from build123d import *

# Parameters (mm, degrees)
F0_W      = 76.2
F0_H      = 76.2
F1_DEPTH  = 76.2
F2_W      = 49.722627
F2_H      = 47.354873
F3_DEPTH  = 25.4
F4_W      = 31.569913
F4_H      = 34.332275
F5_DEPTH  = 50.8
F6_W      = 22.098936
F6_H      = 25.650553
F7_DEPTH  = 154.178
F8_W      = 5.524732
F8_H      = 5.524733
F9_DEPTH  = 171.45
F10_W     = 11.54276
F10_H     = 13.466537
F11_DEPTH = 96.774


with BuildPart() as f1:
    # F0 (on Front) → F1 (new body)
    with BuildSketch(Plane.XZ):
        with Locations((-38.1, 38.1)):
            Rectangle(F0_W, F0_H)
    extrude(amount=F1_DEPTH)

    # F2 (on Top) → F3 (join)
    with BuildSketch(Plane.XY):
        with Locations((-39.363734, -40.251642)):
            Rectangle(F2_W, F2_H)
    extrude(amount=-F3_DEPTH)

    # F4 (on Top) → F5 (join)
    with BuildSketch(Plane.XY):
        with Locations((-40.350295, -40.054333)):
            Rectangle(F4_W, F4_H)
    extrude(amount=-F5_DEPTH)

    # F6 (on Top) → F7 (join)
    with BuildSketch(Plane.XY):
        with Locations((-40.547609, -39.857018)):
            Rectangle(F6_W, F6_H)
    extrude(amount=-F7_DEPTH)

    # F8 (on Top) → F9 (join)
    with BuildSketch(Plane.XY):
        with Locations((-40.547609, -40.251643)):
            Rectangle(F8_W, F8_H)
    extrude(amount=-F9_DEPTH)

    # F10 (on Front) → F11 (cut)
    with BuildSketch(Plane.XZ):
        with Locations((-39.91868, -132.913097)):
            Rectangle(F10_W, F10_H)
    extrude(amount=F11_DEPTH, mode=Mode.SUBTRACT)


solid = f1.part
Verification items for the finished model (mm, model axes). A direction names the side the tool comes from. Give positions to 0.01 mm unless a question says otherwise; leave off trailing zeros. Loops run counter-clockwise (first coordinate to the right, second up) from the corner with the lowest first, then second, coordinate; pieces in that order, holes last.
1. Tool access check on faces 1 (the flat face through (-41, -57.22, -38)), 2 (the flat face through (-41, -22.888, -38)), 3 (the flat face through (-45.69, -40, -133)), 4 (the flat face through (-24.565, -40, -38)). Record the directions out of +Z, -Z, +X, -X, +Y, -Y that give a thin tool (end or side, any length) a straight path to the whole face; none if there is none.
Derived:
face 1: -Z, +X, -X, -Y
face 2: -Z, +X, -X, +Y
face 3: +Y, -Y
face 4: -Z, +X, +Y, -Y
2. Cross-section at A-A on z = -132. Record the cut outline in (x, y).
Derived:
outline: (-51.6, -52.68) - (-45.69, -52.68) - (-45.69, -27.03) - (-51.6, -27.03) - close; (-34.15, -52.68) - (-29.5, -52.68) - (-29.5, -27.03) - (-34.15, -27.03) - close
3. Cross-section at D-D on z = -60. Record the cut outline in (x, y).
Derived:
outline: (-51.6, -52.68) - (-29.5, -52.68) - (-29.5, -27.03) - (-51.6, -27.03) - close
4. Go/stop test with flat-tipped pins: P1, Ø15, axis at y = -43.5, z = -130, coming from the +X side; P2, Ø7.5, axis at y = -44, z = -42.5, coming from the -X side; P3, Ø12.5, axis at y = -31, z = -17, coming from the -X side; P4, Ø12, axis at y = -17, z = -126, coming from the +X side. Record where each tip stops, or that it passes through.
Derived:
P1: stops at x = -29.5
P2: stops at x = -56.14
P3: stops at x = -64.23
P4: passes through
5. Material ranges on probe 1 along Z at (x, y) = (-39, -38.5); probe 2 along Z at (x, y) = (-8.5, -6.5); probe 3 along Z at (x, y) = (-29, -20), recorded low to high.
Derived:
probe 1: z = -171.45 to -139.65, -126.18 to 76.2
probe 2: z = 0 to 76.2
probe 3: z = -25.4 to 76.2
6. Release check for a two-part mould opening along Z. For faces 5 (the flat face through (-64.225, -41, -13)), 6 (the flat face through (-39, -38, 76.2)), 7 (the flat face through (-40, -40, -139.646)) record: +Z half, -Z half, draft (parallel to the pull), parting line (faces both ways), or undercut.
Derived:
face 5: draft
face 6: +Z half
face 7: undercut
7. Cross-section at C-C on x = -18. Record the cut outline in (y, z), and give its area (3 significant figures).
Derived:
outline: (-76.2, 0) - (-63.93, 0) - (-63.93, -25.4) - (-16.57, -25.4) - (-16.57, 0) - (0, 0) - (0, 76.2) - (-76.2, 76.2) - close
area: 7,010 mm2
8. Cross-section at B-B on y = -30.5. Record the cut outline in (x, z).
Derived:
outline: (-76.2, 0) - (-64.23, 0) - (-64.23, -25.4) - (-56.14, -25.4) - (-56.14, -50.8) - (-51.6, -50.8) - (-51.6, -154.18) - (-29.5, -154.18) - (-29.5, -50.8) - (-24.57, -50.8) - (-24.57, -25.4) - (-14.5, -25.4) - (-14.5, 0) - (0, 0) - (0, 76.2) - (-76.2, 76.2) - close; hole (-45.69, -139.65) - (-34.15, -139.65) - (-34.15, -126.18) - (-45.69, -126.18) - close
